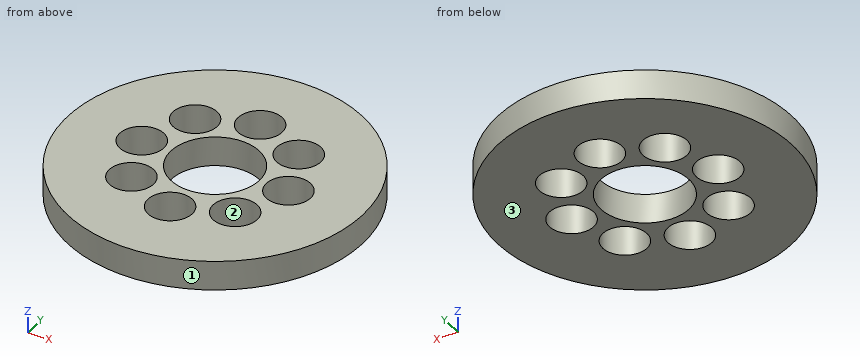
from build123d import *

# Parameters (mm, degrees)
F0_R      = 15.875
F0_R_2    = 4.7625
F1_DEPTH  = 3.175
F3_DEPTH  = 6.35
F4_R      = 15.875
F4_R_2    = 4.7625
F5_DEPTH  = 3.175
F6_R      = 2.38125
F7_DEPTH  = 25.4
F8_R      = 2.38125
F8_R_2    = 1.5875
F9_DEPTH  = 25.4
F10_DEPTH = 3.175
F11_DEPTH = 6.35


with BuildPart() as f1:
    # F0 (on Top) → F1 (new body)
    with BuildSketch(Plane.XY):
        Circle(F0_R)
        Circle(F0_R_2, mode=Mode.SUBTRACT)
    extrude(amount=F1_DEPTH)


with BuildPart() as f3:
    # F2 (on face) → F3 (new body)
    with BuildSketch(Plane.XY.offset(3.175)):
        with BuildLine():
            ThreePointArc((-2.38125, 5.1952741446), (0, 5.715), (2.38125, 5.1952741446))
            Line((2.38125, 5.1952741446), (2.38125, 6.35))
            Line((2.38125, 6.35), (-2.38125, 6.35))
            Line((-2.38125, 6.35), (-2.38125, 5.1952741446))
        make_face()
        with BuildLine():
            Line((2.38125, -6.35), (2.38125, -5.1952741446))
            ThreePointArc((2.38125, -5.1952741446), (0, -5.715), (-2.38125, -5.1952741446))
            Line((-2.38125, -5.1952741446), (-2.38125, -6.35))
            Line((-2.38125, -6.35), (2.38125, -6.35))
        make_face()
        with BuildLine():
            ThreePointArc((-2.38125, 4.1244459855), (0, 4.7625), (2.38125, 4.1244459855))
            Line((2.38125, 4.1244459855), (2.38125, 5.1952741446))
            ThreePointArc((2.38125, 5.1952741446), (0, 5.715), (-2.38125, 5.1952741446))
            Line((-2.38125, 5.1952741446), (-2.38125, 4.1244459855))
        make_face()
        with BuildLine():
            ThreePointArc((2.38125, 4.1244459855), (3.3675960454, 3.3675960454), (4.1244459855, 2.38125))
            Line((4.1244459855, 2.38125), (5.1952741446, 2.38125))
            ThreePointArc((5.1952741446, 2.38125), (4.0411152545, 4.0411152545), (2.38125, 5.1952741446))
            Line((2.38125, 5.1952741446), (2.38125, 4.1244459855))
        make_face()
        with BuildLine():
            Line((2.38125, -5.1952741446), (2.38125, -4.1244459855))
            ThreePointArc((2.38125, -4.1244459855), (0, -4.7625), (-2.38125, -4.1244459855))
            Line((-2.38125, -4.1244459855), (-2.38125, -5.1952741446))
            ThreePointArc((-2.38125, -5.1952741446), (0, -5.715), (2.38125, -5.1952741446))
        make_face()
        with BuildLine():
            Line((-2.38125, -5.1952741446), (-2.38125, -4.1244459855))
            ThreePointArc((-2.38125, -4.1244459855), (-3.3675960454, -3.3675960454), (-4.1244459855, -2.38125))
            Line((-4.1244459855, -2.38125), (-5.1952741446, -2.38125))
            ThreePointArc((-5.1952741446, -2.38125), (-4.0411152545, -4.0411152545), (-2.38125, -5.1952741446))
        make_face()
        with BuildLine():
            ThreePointArc((-4.1244459855, -2.38125), (-4.7625, 0), (-4.1244459855, 2.38125))
            Line((-4.1244459855, 2.38125), (-5.1952741446, 2.38125))
            ThreePointArc((-5.1952741446, 2.38125), (-5.715, 0), (-5.1952741446, -2.38125))
            Line((-5.1952741446, -2.38125), (-4.1244459855, -2.38125))
        make_face()
        with BuildLine():
            ThreePointArc((-4.1244459855, 2.38125), (-3.3675960454, 3.3675960454), (-2.38125, 4.1244459855))
            Line((-2.38125, 4.1244459855), (-2.38125, 5.1952741446))
            ThreePointArc((-2.38125, 5.1952741446), (-4.0411152545, 4.0411152545), (-5.1952741446, 2.38125))
            Line((-5.1952741446, 2.38125), (-4.1244459855, 2.38125))
        make_face()
        with BuildLine():
            ThreePointArc((-5.1952741446, -2.38125), (-5.715, 0), (-5.1952741446, 2.38125))
            Line((-5.1952741446, 2.38125), (-6.35, 2.38125))
            Line((-6.35, 2.38125), (-6.35, -2.38125))
            Line((-6.35, -2.38125), (-5.1952741446, -2.38125))
        make_face()
    extrude(amount=F3_DEPTH)



with BuildPart() as f3b:
    # F2 (on face) → F3, piece 2 (new body)
    with BuildSketch(Plane.XY.offset(3.175)):
        with BuildLine():
            Line((6.35, 2.38125), (5.1952741446, 2.38125))
            ThreePointArc((5.1952741446, 2.38125), (5.5835569638, 1.2186536144), (5.715, 0))
            ThreePointArc((5.715, 0), (5.5835569638, -1.2186536144), (5.1952741446, -2.38125))
            Line((5.1952741446, -2.38125), (6.35, -2.38125))
            Line((6.35, -2.38125), (6.35, 2.38125))
        make_face()
    extrude(amount=F3_DEPTH)


with BuildPart() as f3_1:
    add(f3.part)

    add(f3b.part)  # F5 merges F3b
    # F4 (on face) → F5 (join)
    with BuildSketch(Plane.XY.offset(9.525)):
        Circle(F4_R)
        Circle(F4_R_2, mode=Mode.SUBTRACT)
    extrude(amount=F5_DEPTH)


with BuildPart() as f7_tool:
    # F6 (on face) → F7 (new body)
    with BuildSketch(Plane.XY.offset(12.7)):
        with Locations((-5.6126600757, 5.6126600757)):
            Circle(F6_R)
        with Locations((5.6126600757, -5.6126600757)):
            Circle(F6_R)
        with Locations((0, 7.9375)):
            Circle(F6_R)
        with Locations((5.6126600757, 5.6126600757)):
            Circle(F6_R)
        with Locations((7.9375, 0)):
            Circle(F6_R)
        with Locations((0, -7.9375)):
            Circle(F6_R)
        with Locations((-5.6126600757, -5.6126600757)):
            Circle(F6_R)
        with Locations((-7.9375, 0)):
            Circle(F6_R)
    extrude(amount=-F7_DEPTH)


with BuildPart() as f1_1:
    add(f1.part)

    # F7: cut by f7_tool
    add(f7_tool.part, mode=Mode.SUBTRACT)

    # F8 (on face) → F9 (cut)
    with BuildSketch(Plane(origin=(0, 0, 0), x_dir=(1, 0, 0), z_dir=(0, 0, -1))):
        with Locations((0, 7.9375)):
            Circle(F8_R)
        with Locations((0, 7.9375)):
            Circle(F8_R_2, mode=Mode.SUBTRACT)
        with Locations((5.6126600757, 5.6126600757)):
            Circle(F8_R)
        with Locations((5.6126600757, 5.6126600757)):
            Circle(F8_R_2, mode=Mode.SUBTRACT)
        with Locations((7.9375, 0)):
            Circle(F8_R)
        with Locations((7.9375, 0)):
            Circle(F8_R_2, mode=Mode.SUBTRACT)
        with Locations((5.6126600757, -5.6126600757)):
            Circle(F8_R)
        with Locations((5.6126600757, -5.6126600757)):
            Circle(F8_R_2, mode=Mode.SUBTRACT)
        with Locations((0, -7.9375)):
            Circle(F8_R)
        with Locations((0, -7.9375)):
            Circle(F8_R_2, mode=Mode.SUBTRACT)
        with Locations((-5.6126600757, -5.6126600757)):
            Circle(F8_R)
        with Locations((-5.6126600757, -5.6126600757)):
            Circle(F8_R_2, mode=Mode.SUBTRACT)
        with Locations((-7.9375, 0)):
            Circle(F8_R)
        with Locations((-7.9375, 0)):
            Circle(F8_R_2, mode=Mode.SUBTRACT)
        with Locations((-5.6126600757, 5.6126600757)):
            Circle(F8_R)
        with Locations((-5.6126600757, 5.6126600757)):
            Circle(F8_R_2, mode=Mode.SUBTRACT)
        with Locations((7.9375, 0)):
            Circle(F8_R_2)
        with Locations((5.6126600757, -5.6126600757)):
            Circle(F8_R_2)
        with Locations((0, -7.9375)):
            Circle(F8_R_2)
        with Locations((-5.6126600757, -5.6126600757)):
            Circle(F8_R_2)
        with Locations((-7.9375, 0)):
            Circle(F8_R_2)
        with Locations((-5.6126600757, 5.6126600757)):
            Circle(F8_R_2)
        with Locations((0, 7.9375)):
            Circle(F8_R_2)
        with Locations((5.6126600757, 5.6126600757)):
            Circle(F8_R_2)
    extrude(amount=-F9_DEPTH, mode=Mode.SUBTRACT)


with BuildPart() as f3_2:
    add(f3_1.part)

    # F7: cut by f7_tool
    add(f7_tool.part, mode=Mode.SUBTRACT)

    # F10 (cut): a face of the model
    f10_faces = [f3_2.faces().sort_by_distance(p)[0] for p in [
        (-15.4259871939, 0, 12.7),
    ]]
    extrude(f10_faces, amount=-F10_DEPTH, mode=Mode.SUBTRACT)

    # F11 (cut): faces of the model
    f11_faces = [f3_2.faces().sort_by_distance(p)[0] for p in [
        (5.820119134, -1.8463906572, 9.525),
        (-3.8074982703, -3.8074982703, 9.525),
        (5.820119134, 1.8463906572, 9.525),
    ]]
    extrude(f11_faces, amount=-F11_DEPTH, mode=Mode.SUBTRACT)


solid = f1_1.part
Part model, mm, in its own coordinate system. Face numbers are marked on the shaded views. Coordinates: 2 decimals unless noted, no trailing zeros. Order: outer loops, then holes, each group sorted by start corner. A loop starts at its lowest first (then second) coordinate and runs counter-clockwise, first axis right, second up.
(1) Slice it at C-C, the plane z = 1.5. State how many separate pieces and enclosed holes the cut face has, and give its area (3 significant figures).
Check sheet entries:
separate pieces: 1
enclosed holes: 9
area: 578 mm2
(2) Pin check, flat tips, straight feed: pin 1 Ø4.5 at (x, y) = (0, 7.94) entering from +Z; pin 2 Ø1.5 at (x, z) = (7.5, 1) entering from -Y. Stop position of each tip, or through.
Check sheet entries:
pin 1: passes through
pin 2: stops at y = -14.37
(3) Pull direction Y, two halves, no side cores. Call the marked faces 1, 2 and 3: pulls with the +Y half, pulls with the -Y half, needs draft (parallel to the pull), parting line crosses it, or undercut.
Check sheet entries:
face 1: parting line crosses it
face 2: undercut
face 3: needs draft
(4) Slice it at B-B, the plane y = 1.5. Write the cut outline in (x, z) (3 decimals), and give its area (3 significant figures).
Check sheet entries:
outline: (-15.804, 0) - (-9.787, 0) - (-9.787, 3.175) - (-15.804, 3.175) - close; (-6.088, 0) - (-4.52, 0) - (-4.52, 3.175) - (-6.088, 3.175) - close; (4.52, 0) - (6.088, 0) - (6.088, 3.175) - (4.52, 3.175) - close; (9.787, 0) - (15.804, 0) - (15.804, 3.175) - (9.787, 3.175) - close
area: 48.2 mm2
(5) Slice it at D-D, the plane y = 8.5. Write the cut outline in (x, z) (3 decimals).
Check sheet entries:
outline: (-13.408, 0) - (-2.314, 0) - (-2.314, 3.175) - (-13.408, 3.175) - close; (2.314, 0) - (13.408, 0) - (13.408, 3.175) - (2.314, 3.175) - close
(6) Slice it at A-A, the plane x = 0. Write the cut outline in (y, z) (1 decimal), and give its area (3 significant figures).
Check sheet entries:
outline: (-15.9, 0) - (-10.3, 0) - (-10.3, 3.2) - (-15.9, 3.2) - close; (-5.6, 0) - (-4.8, 0) - (-4.8, 3.2) - (-5.6, 3.2) - close; (4.8, 0) - (5.6, 0) - (5.6, 3.2) - (4.8, 3.2) - close; (10.3, 0) - (15.9, 0) - (15.9, 3.2) - (10.3, 3.2) - close
area: 40.3 mm2
(7) Probe L1, parallel to Y at x = 0, z = 2.6 (1 decimal); L2, parallel to X at y = -5.5, z = 1.3; L3, parallel to X at y = 3.5, z = 2.1. List the from-to ranges inside material, lowest first.
Check sheet entries:
L1: y = -15.9 to -10.3, -5.6 to -4.8, 4.8 to 5.6, 10.3 to 15.9
L2: x = -14.89 to -7.99, -3.23 to 3.23, 7.99 to 14.89
L3: x = -15.48 to -6.71, -4.51 to -3.23, 3.23 to 4.51, 6.71 to 15.48
